Here's the drawing with two shaded views (mm, measured from the low corner). I have some questions. Coordinates: 2 decimals unless noted, no trailing zeros. Loops run counter-clockwise (first coordinate to the right, second up) from the corner with the lowest first, then second, coordinate; pieces in that order, holes last. Notation, with made-up numbers: (9, -15.5) - (47, -15.5) arc R24 ccw to (47, 10.5) - close; hole circle Ø11 at (-33, 87). An arc over 180 degrees is marked (long way). Use a Markdown table: item, result.
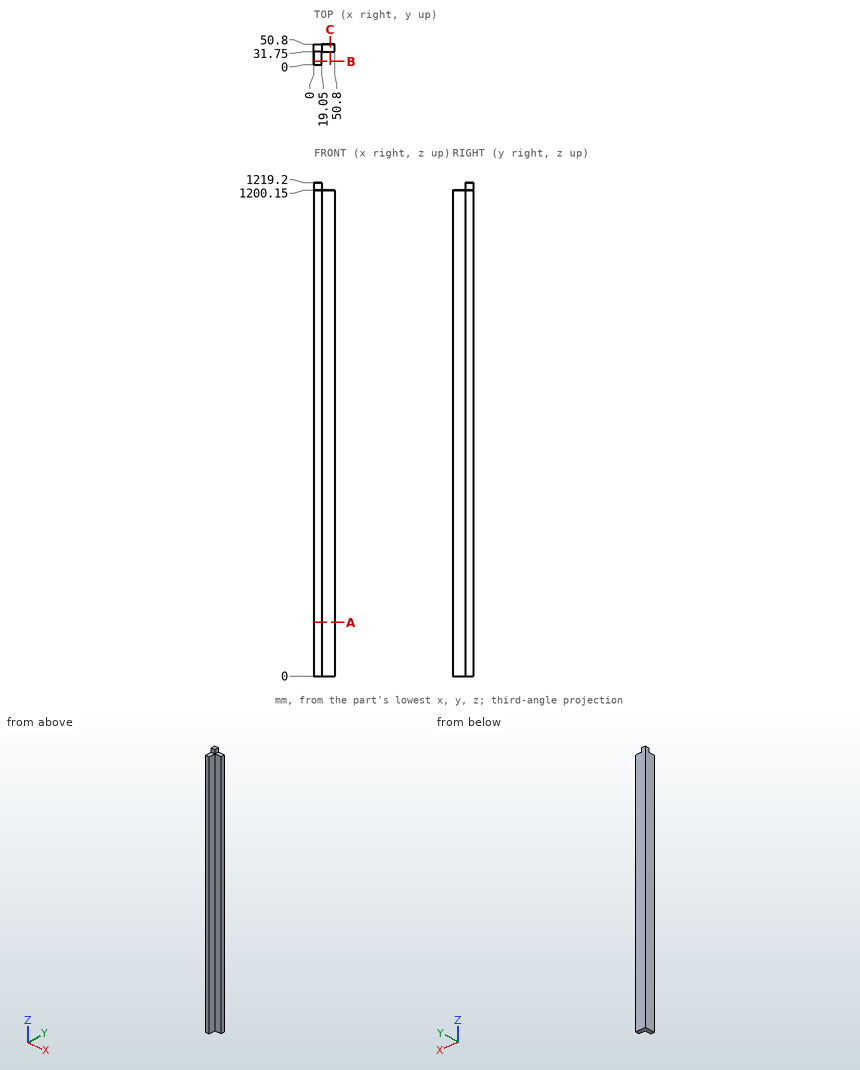
Q1. I want a section at A-A, the plane z = 132.5. Write out the boundary of the cut face in (x, y), then the cut area to 3 significant figures.
Check values:
| item | result |
|---|---|
| outline | (0, 0) - (19.05, 0) - (19.05, 31.75) - (50.8, 31.75) - (50.8, 50.8) - (0, 50.8) - close |
| area | 1,570 mm^2 |
Q2. I want a section at C-C, the plane x = 40. Write out the boundary of the cut face in (y, z).
Check values:
| item | result |
|---|---|
| outline | (31.75, 0) - (50.8, 0) - (50.8, 1200.15) - (31.75, 1200.15) - close |
Q3. Will these pins go through, and if not, where does the flat tip stop? P1, Ø5.5, axis at y = 38, z = 1208, coming from the +X side; P2, Ø1.5, axis at y = 19, z = 402, coming from the +X side; P3, Ø8, axis at x = 35, z = 1084, coming from the -Y side.
Check values:
| item | result |
|---|---|
| P1 | x = 19.05 |
| P2 | x = 19.05 |
| P3 | y = 31.75 |
Q4. Please list where these lines run through material, in increasing order: L1, parallel to Y at x = 30, z = 1137.5; L2, parallel to X at y = 22, z = 922.5; L3, parallel to Z at x = 11, y = 6. Write a range as from..to.
Check values:
| item | result |
|---|---|
| L1 | 31.75..50.8 |
| L2 | 0..19.05 |
| L3 | 0..1200.15 |
Q5. I want a section at B-B, the plane y = 8. Write out the boundary of the cut face in (x, z), then the cut area to 3 significant figures.
Check values:
| item | result |
|---|---|
| outline | (0, 0) - (19.05, 0) - (19.05, 1200.15) - (0, 1200.15) - close |
| area | 22,900 mm^2 |
